from build123d import *

# Parameters (mm, degrees)
F0_R     = 4.25
F1_DEPTH = 3.3
F2_R     = 2.5
F3_DEPTH = 20
F4_W     = 12.181458
F4_H     = 1.3
F5_DEPTH = 1.2
F6_R     = 1


with BuildPart() as f1:
    # F0 (on Top) → F1 (new body)
    with BuildSketch(Plane.XY):
        Circle(F0_R)
    extrude(amount=F1_DEPTH)

    # F2 (on face) → F3 (join)
    with BuildSketch(Plane(origin=(0, 0, 0), x_dir=(1, 0, 0), z_dir=(0, 0, -1))):
        Circle(F2_R)
    extrude(amount=F3_DEPTH)

    # F4 (on face) → F5 (cut)
    with BuildSketch(Plane.XY.offset(3.3)):
        Rectangle(F4_W, F4_H)
    extrude(amount=-F5_DEPTH, mode=Mode.SUBTRACT)

    # F6
    f6_edges = [f1.edges().sort_by_distance(p)[0] for p in [
        (0, -4.25, 3.3),
        (0, 4.25, 3.3),
    ]]
    fillet(f6_edges, radius=F6_R)


solid = f1.part
Part model, mm, in its own coordinate system. A direction names the side the tool comes from. Give positions to 0.01 mm unless a question says otherwise; leave off trailing zeros. Loops run counter-clockwise (first coordinate to the right, second up) from the corner with the lowest first, then second, coordinate; pieces in that order, holes last.
(1) Pull direction Y, two halves, no side cores. Call faces 1 (the flat face through (2, -2, 0)), 2 (the cylindrical face through (4.054, 1.277, 1.134)), 3 (the flat face through (0, 0, 2.1)), 4 (the flat face through (0, -0.65, 3)): pulls with the +Y half, pulls with the -Y half, needs draft (parallel to the pull), parting line crosses it, or undercut.
Return value:
face 1: needs draft
face 2: parting line crosses it
face 3: undercut
face 4: undercut
(2) Band-saw the part on A-A (x = 0). Write the cut outline in (y, z).
Return value:
outline: (-4.25, 0) - (-2.5, 0) - (-2.5, -20) - (2.5, -20) - (2.5, 0) - (4.25, 0) - (4.25, 2.3) arc R1 ccw to (3.25, 3.3) - (0.65, 3.3) - (0.65, 2.1) - (-0.65, 2.1) - (-0.65, 3.3) - (-3.25, 3.3) arc R1 ccw to (-4.25, 2.3) - close
(3) Drill centre lines: line 1 along Z through (x, y) = (3.75, 0.5); line 2 along Z through (x, y) = (-0.5, 3.25); line 3 along X through (y, z) = (0, -14.5). Where is each one in solid material? Low to high.
Return value:
line 1: z = 0 to 2.1
line 2: z = 0 to 3.3
line 3: x = -2.5 to 2.5
(4) Pin check, flat tips, straight feed: pin 1 (4 mm diameter, centred on x = -1.5, y = 3, fed in from +Z); pin 2 (1 mm diameter, centred on x = -3.5, y = 2.5, fed in from -Z); pin 3 (0.7 mm diameter, centred on x = 0.5, y = 0, fed in from +Z); pin 4 (1.3 mm diameter, centred on x = 2, z = 3, fed in from +Y). Stop position of each tip, or through.
Return value:
pin 1: stops at z = 3.3
pin 2: stops at z = 0
pin 3: stops at z = 2.1
pin 4: stops at y = 3.93
(5) Band-saw the part on B-B (y = 0). Write the cut outline in (x, z), and give its area (3 significant figures).
Return value:
outline: (-4.25, 0) - (-2.5, 0) - (-2.5, -20) - (2.5, -20) - (2.5, 0) - (4.25, 0) - (4.25, 2.1) - (-4.25, 2.1) - close
area: 118 mm2
(6) Band-saw the part on C-C (z = -8.75). Write the cut outline in (x, y).
Return value:
outline: circle Ø5 at (0, 0)
(7) 3-axis set-ups, long thin cutter, end or side, ignore diameter. For faces 5 (the flat face through (0, 2, 3.3)), 6 (the flat face through (0, 0.65, 3)), 7 (the cylindrical face through (-0.54, 2.44, -9.86)): which of +Z, -Z, +X, -X, +Y, -Y reach the whole face in a straight line?
Return value:
face 5: +Z, +X, -X, +Y, -Y
face 6: +Z, +X, -X
face 7: -Z
